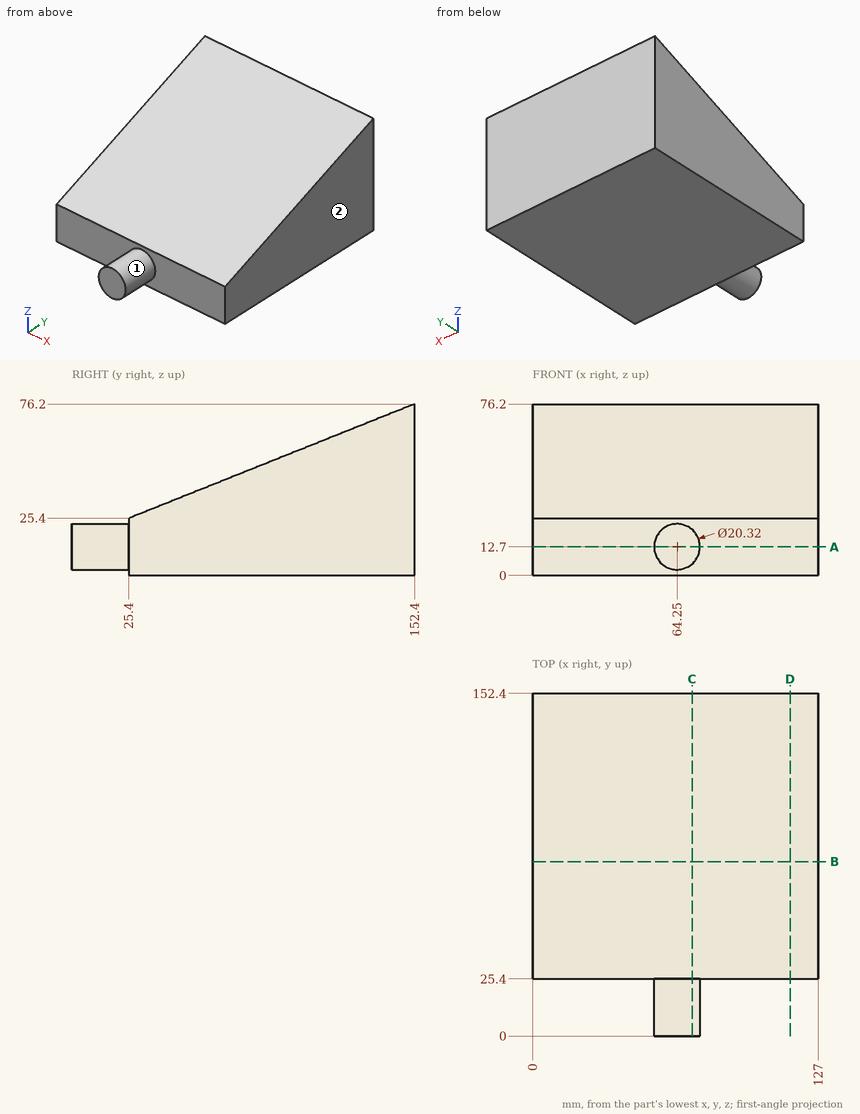
Could you check a few things on this drawing? It's one solid part, dimensions in mm from its lowest x, y, z. A direction names the side the tool comes from. Round coordinates to 2 decimals unless told otherwise and drop trailing zeros. Write each loop counter-clockwise with the first axis right and the second up, starting at its lowest first coordinate (ties: lowest second). Pieces come first, ordered by that corner, then holes.
Q1. If we section it at C-C on x = 71: Write out the boundary of the cut face in (y, z).
Q2. If we section it at B-B on y = 77.5: Write out the boundary of the cut face in (x, z).
Q3. Will these pins go through, and if not, where does the flat tip stop? P1, Ø7.5, axis at x = 65, z = 15, coming from the -Y side; P2, Ø10, axis at x = 51.5, y = 113, coming from the +Z side.
Q4. Which directions (+Z, -Z, +X, -X, +Y, -Y) give clear straight access to the entire face, cutting with the end or side of a thin tool? Please do the marked faces 1 and 2.
Q5. If we section it at D-D on x = 114.5: Write out the boundary of the cut face in (y, z), plus the area to 3 significant figures.
Q6. If we section it at A-A on z = 12.7: Write out the boundary of the cut face in (x, y), plus the area to 3 significant figures.
Q7. Please list where these lines run through material, in increasing order: probe 1 along Y at (x, z) = (26, 3.5); probe 2 along Z at (x, y) = (48.5, 87); probe 3 along Z at (x, y) = (90, 58).
Answer below:
1. outline: (0, 5.11) - (25.4, 5.11) - (25.4, 0) - (152.4, 0) - (152.4, 76.2) - (25.4, 25.4) - (25.4, 20.29) - (0, 20.29) - close
2. outline: (0, 0) - (127, 0) - (127, 46.24) - (0, 46.24) - close
3. P1: stops at y = 0
3. P2: stops at z = 62.44
4. face 1: -Y
4. face 2: +Z, -Z, +X, +Y, -Y
5. outline: (25.4, 0) - (152.4, 0) - (152.4, 76.2) - (25.4, 25.4) - close
5. area: 6,450 mm2
6. outline: (0, 25.4) - (54.09, 25.4) - (54.09, 0) - (74.41, 0) - (74.41, 25.4) - (127, 25.4) - (127, 152.4) - (0, 152.4) - close
6. area: 16,600 mm2
7. probe 1: y = 25.4 to 152.4
7. probe 2: z = 0 to 50.04
7. probe 3: z = 0 to 38.44
